```python
from build123d import *

# Parameters (mm, degrees)
F0_W            = 262
F0_H            = 139.5
F1_DEPTH        = 3
F3_DEPTH        = 3.001
F5_D            = 3.3
F5_CSINK_D      = 6.72
F5_CSINK_ANGLE  = 90
F7_D            = 3.3
F7_CSINK_D      = 6.72
F7_CSINK_ANGLE  = 90
F8_DEPTH        = 3.001
F10_D           = 4.4
F10_CSINK_D     = 8.96
F10_CSINK_ANGLE = 90


with BuildPart() as f1:
    # F0 (on Front) → F1 (new body)
    with BuildSketch(Plane.XZ):
        with Locations((131, 69.75)):
            Rectangle(F0_W, F0_H)
    extrude(amount=F1_DEPTH)

    # F2 (on face) → F3 (cut, through all)
    with BuildSketch(Plane(origin=(0, 0, 0), x_dir=(-1, 0, 0), z_dir=(0, 1, 0))):
        with BuildLine():
            Line((-30, 111), (-43, 111))
            ThreePointArc((-43, 111), (-44.4142135624, 110.4142135624), (-45, 109))
            Line((-45, 109), (-45, 26))
            ThreePointArc((-45, 26), (-44.4142135624, 24.5857864376), (-43, 24))
            Line((-43, 24), (-30, 24))
            Line((-30, 24), (-30, 111))
        make_face()
        with BuildLine():
            Line((-17, 111), (-30, 111))
            Line((-30, 111), (-30, 24))
            Line((-30, 24), (-17, 24))
            ThreePointArc((-17, 24), (-15.5857864376, 24.5857864376), (-15, 26))
            Line((-15, 26), (-15, 109))
            ThreePointArc((-15, 109), (-15.5857864376, 110.4142135624), (-17, 111))
        make_face()
    extrude(amount=-F3_DEPTH, mode=Mode.SUBTRACT)

    # F5 (through all)
    with Locations(Plane(origin=(0, 0, 0), x_dir=(-1, 0, 0), z_dir=(0, 1, 0))):
        with Locations((-30, 119), (-30, 16)):
            CounterSinkHole(F5_D / 2, F5_CSINK_D / 2, counter_sink_angle=F5_CSINK_ANGLE)

    # F7 (through all)
    with Locations(Plane(origin=(0, 0, 0), x_dir=(-1, 0, 0), z_dir=(0, 1, 0))):
        with Locations((-217.86, 113), (-200.08, 113), (-182.3, 113), (-164.52, 113), (-146.74, 113), (-128.96, 113), (-111.18, 113), (-93.4, 113), (-93.4, 21), (-111.18, 21), (-146.74, 21), (-164.52, 21), (-128.96, 21), (-182.3, 21), (-217.86, 21), (-200.08, 21)):
            CounterSinkHole(F7_D / 2, F7_CSINK_D / 2, counter_sink_angle=F7_CSINK_ANGLE)

    # F6 (on face) → F8 (cut, through all)
    with BuildSketch(Plane(origin=(0, 0, 0), x_dir=(-1, 0, 0), z_dir=(0, 1, 0))):
        with BuildLine():
            Line((-98.9, 27), (-87.9, 27))
            ThreePointArc((-87.9, 27), (-86.4857864376, 27.5857864376), (-85.9, 29))
            Line((-85.9, 29), (-85.9, 105))
            ThreePointArc((-85.9, 105), (-86.4857864376, 106.4142135624), (-87.9, 107))
            Line((-87.9, 107), (-98.9, 107))
            ThreePointArc((-98.9, 107), (-100.3142135624, 106.4142135624), (-100.9, 105))
            Line((-100.9, 105), (-100.9, 29))
            ThreePointArc((-100.9, 29), (-100.3142135624, 27.5857864376), (-98.9, 27))
        make_face()
        with BuildLine():
            ThreePointArc((-103.68, 105), (-104.2657864376, 106.4142135624), (-105.68, 107))
            Line((-105.68, 107), (-116.68, 107))
            ThreePointArc((-116.68, 107), (-118.0942135624, 106.4142135624), (-118.68, 105))
            Line((-118.68, 105), (-118.68, 29))
            ThreePointArc((-118.68, 29), (-118.0942135624, 27.5857864376), (-116.68, 27))
            Line((-116.68, 27), (-105.68, 27))
            ThreePointArc((-105.68, 27), (-104.2657864376, 27.5857864376), (-103.68, 29))
            Line((-103.68, 29), (-103.68, 105))
        make_face()
        with BuildLine():
            ThreePointArc((-121.46, 105), (-122.0457864376, 106.4142135624), (-123.46, 107))
            Line((-123.46, 107), (-134.46, 107))
            ThreePointArc((-134.46, 107), (-135.8742135624, 106.4142135624), (-136.46, 105))
            Line((-136.46, 105), (-136.46, 29))
            ThreePointArc((-136.46, 29), (-135.8742135624, 27.5857864376), (-134.46, 27))
            Line((-134.46, 27), (-123.46, 27))
            ThreePointArc((-123.46, 27), (-122.0457864376, 27.5857864376), (-121.46, 29))
            Line((-121.46, 29), (-121.46, 105))
        make_face()
        with BuildLine():
            ThreePointArc((-139.24, 105), (-139.8257864376, 106.4142135624), (-141.24, 107))
            Line((-141.24, 107), (-152.24, 107))
            ThreePointArc((-152.24, 107), (-153.6542135624, 106.4142135624), (-154.24, 105))
            Line((-154.24, 105), (-154.24, 29))
            ThreePointArc((-154.24, 29), (-153.6542135624, 27.5857864376), (-152.24, 27))
            Line((-152.24, 27), (-141.24, 27))
            ThreePointArc((-141.24, 27), (-139.8257864376, 27.5857864376), (-139.24, 29))
            Line((-139.24, 29), (-139.24, 105))
        make_face()
        with BuildLine():
            ThreePointArc((-157.02, 105), (-157.6057864376, 106.4142135624), (-159.02, 107))
            Line((-159.02, 107), (-170.02, 107))
            ThreePointArc((-170.02, 107), (-171.4342135624, 106.4142135624), (-172.02, 105))
            Line((-172.02, 105), (-172.02, 29))
            ThreePointArc((-172.02, 29), (-171.4342135624, 27.5857864376), (-170.02, 27))
            Line((-170.02, 27), (-159.02, 27))
            ThreePointArc((-159.02, 27), (-157.6057864376, 27.5857864376), (-157.02, 29))
            Line((-157.02, 29), (-157.02, 105))
        make_face()
        with BuildLine():
            ThreePointArc((-174.8, 105), (-175.3857864376, 106.4142135624), (-176.8, 107))
            Line((-176.8, 107), (-187.8, 107))
            ThreePointArc((-187.8, 107), (-189.2142135624, 106.4142135624), (-189.8, 105))
            Line((-189.8, 105), (-189.8, 29))
            ThreePointArc((-189.8, 29), (-189.2142135624, 27.5857864376), (-187.8, 27))
            Line((-187.8, 27), (-176.8, 27))
            ThreePointArc((-176.8, 27), (-175.3857864376, 27.5857864376), (-174.8, 29))
            Line((-174.8, 29), (-174.8, 105))
        make_face()
        with BuildLine():
            ThreePointArc((-192.58, 105), (-193.1657864376, 106.4142135624), (-194.58, 107))
            Line((-194.58, 107), (-205.58, 107))
            ThreePointArc((-205.58, 107), (-206.9942135624, 106.4142135624), (-207.58, 105))
            Line((-207.58, 105), (-207.58, 29))
            ThreePointArc((-207.58, 29), (-206.9942135624, 27.5857864376), (-205.58, 27))
            Line((-205.58, 27), (-194.58, 27))
            ThreePointArc((-194.58, 27), (-193.1657864376, 27.5857864376), (-192.58, 29))
            Line((-192.58, 29), (-192.58, 105))
        make_face()
        with BuildLine():
            ThreePointArc((-210.36, 105), (-210.9457864376, 106.4142135624), (-212.36, 107))
            Line((-212.36, 107), (-223.36, 107))
            ThreePointArc((-223.36, 107), (-224.7742135624, 106.4142135624), (-225.36, 105))
            Line((-225.36, 105), (-225.36, 29))
            ThreePointArc((-225.36, 29), (-224.7742135624, 27.5857864376), (-223.36, 27))
            Line((-223.36, 27), (-212.36, 27))
            ThreePointArc((-212.36, 27), (-210.9457864376, 27.5857864376), (-210.36, 29))
            Line((-210.36, 29), (-210.36, 105))
        make_face()
    extrude(amount=-F8_DEPTH, mode=Mode.SUBTRACT)

    # F10 (through all)
    with Locations(Plane(origin=(0, 0, 0), x_dir=(-1, 0, 0), z_dir=(0, 1, 0))):
        with Locations((-9.5, 124.5), (-238, 129), (-54, 129), (-238, 9.5), (-54, 9.5)):
            CounterSinkHole(F10_D / 2, F10_CSINK_D / 2, counter_sink_angle=F10_CSINK_ANGLE)


solid = f1.part
```
The model under review builds one solid part; all positions refer to its coordinate system, in mm. Give positions to 0.01 mm unless a question says otherwise; leave off trailing zeros. Answer as a JSON object with one key per item and string values.
Q1. To check wall thickness, follow line 1 along Z through (x, y) = (111.18, -1.95); line 2 along X through (y, z) = (-2.5, 129); line 3 along Z through (x, y) = (117, -2.3). State the ranges of each line that lie inside material, in increasing order.
Worked out:
{"line 1": "z = 0 to 19.35, 22.65 to 27, 107 to 111.35, 114.65 to 139.5", "line 2": "x = 0 to 51.8, 56.2 to 235.8, 240.2 to 262", "line 3": "z = 0 to 27.03, 106.97 to 139.5"}
Q2. Add section A-A on z = 45.5. Count the separate pieces of the cut face and the enclosed holes in it, plus the area to 3 significant figures.
Worked out:
{"separate pieces": "10", "enclosed holes": "0", "area": "336 mm^2"}
Q3. Mouldability with a two-part tool opening along X and no side actions: class faces 1 (the conical face through (112.1, -1.6, 114.5)), 2 (the flat face through (129, -3, 117)) as +X half, -X half, draft (parallel to the pull), parting line (faces both ways), or undercut.
Worked out:
{"face 1": "undercut", "face 2": "draft"}
